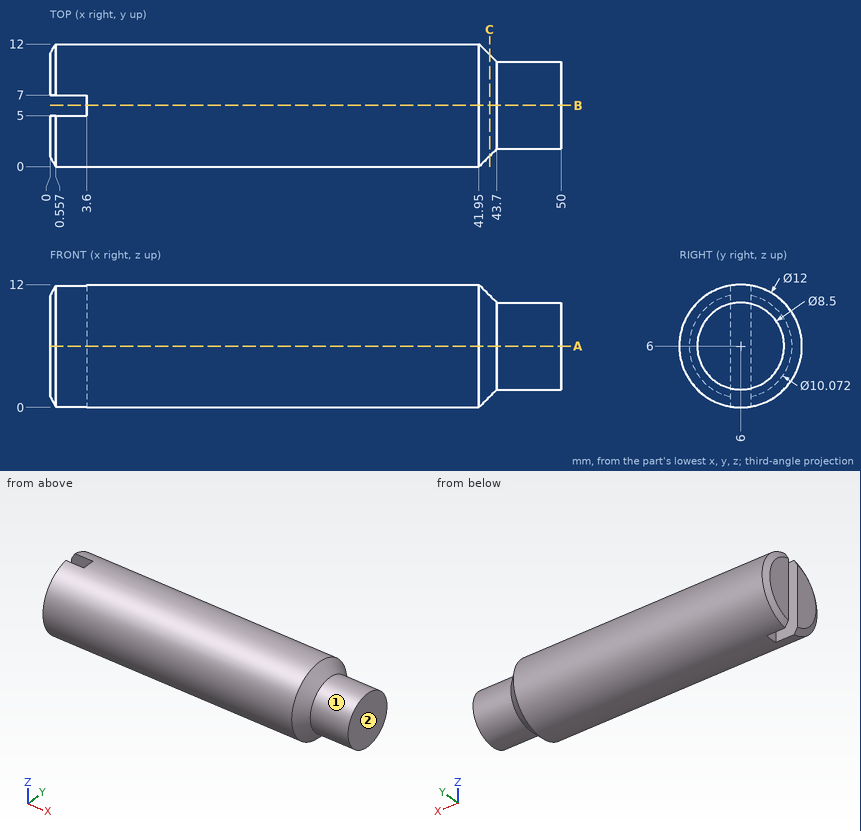
The figure shows three views and two pictorial views of one solid part (mm, origin at its lowest corner). Answer the questions. A direction names the side the tool comes from. Give positions to 0.01 mm unless a question says otherwise; leave off trailing zeros. Order: outer loops, then holes, each group sorted by start corner. A loop starts at its lowest first (then second) coordinate and runs counter-clockwise, first axis right, second up. Notation, with made-up numbers: (72, 28.5) -> (127, 28.5) arc R23 cw to (127, 46.5) -> close; hole circle Ø10 at (84.25, 54). An arc over 180 degrees is marked (long way). Answer as a JSON object with one key per item and string values. Group by question number.
Item 1: The part is cut by section A-A on z = 6. Write down the section's boundary in (x, y).
Item 2: Consider L1, parallel to Z at x = 9.5, y = 5 (1 decimal); L2, parallel to X at y = 5.25, z = 5.25; L3, parallel to Y at x = 10.5, z = 6.25 (1 decimal). Determine where each line is inside the solid, lowest interval first. Write a range as from..to.
Item 3: The part is cut by section C-C on x = 43. Write down the section's boundary in (y, z).
Item 4: A tool of negligible diameter and unlimited length cuts with its end or side. For the marked faces 1 and 2, from which of +Z, -Z, +X, -X, +Y, -Y can it reach the whole face along a straight path? Write none if from no direction.
Item 5: The part is cut by section B-B on y = 6. Write down the section's boundary in (x, z).
Item 6: Flat-ended cylindrical pins translate along their axes: pin 1 (1.1 mm diameter, centred on x = 1, z = 4.5, fed in from -Y); pin 2 (3 mm diameter, centred on x = 2, z = 7, fed in from +Y); pin 3 (1.5 mm diameter, centred on x = 35.5, z = 10.5, fed in from +Y) (1 decimal); pin 4 (2 mm diameter, centred on x = 29, y = 3, fed in from +Z). Find the tip coordinate at first contact, or state that the pin passes through.
Result set:
{
 "1": {"outline": "(0, 0.96) -> (0.56, 0) -> (41.95, 0) -> (43.7, 1.75) -> (50, 1.75) -> (50, 10.25) -> (43.7, 10.25) -> (41.95, 12) -> (0.56, 12) -> (0, 11.04) -> (0, 7) -> (3.6, 7) -> (3.6, 5) -> (0, 5) -> close"},
 "2": {"L1": "0.1..11.9", "L2": "3.6..50", "L3": "0..12"},
 "3": {"outline": "circle Ø9.9 at (6, 6)"},
 "4": {"face 1": "+X", "face 2": "+Z, -Z, +X, +Y, -Y"},
 "5": {"outline": "(3.6, 0) -> (41.95, 0) -> (43.7, 1.75) -> (50, 1.75) -> (50, 10.25) -> (43.7, 10.25) -> (41.95, 12) -> (3.6, 12) -> close"},
 "6": {"pin 1": "y = 0.08", "pin 2": "y = 12", "pin 3": "y = 10.7", "pin 4": "z = 11.66"}
}
